```python
from build123d import *

# Parameters (mm, degrees)
BOSS_EXTRUDE1_DEPTH = 0.127
SKETCH2_R           = 3.3782
CUT_EXTRUDE1_DEPTH  = 124.294763186


with BuildPart() as part:
    # Sketch1 → Boss-Extrude1 (new body)
    with BuildSketch(Plane(origin=(0, 0, 0), x_dir=(1, 0, 0), z_dir=(0, 1, 0))):
        with BuildLine():
            Line((19.05, 44.45), (69.85, 44.45))
            ThreePointArc((69.85, 44.45), (74.340128061, 42.590128061), (76.2, 38.1))
            Line((76.2, 38.1), (76.2, -38.1))
            ThreePointArc((76.2, -38.1), (74.340128061, -42.590128061), (69.85, -44.45))
            Line((69.85, -44.45), (19.05, -44.45))
            Line((19.05, -44.45), (19.05, -60.325))
            Line((19.05, -60.325), (15.875, -60.325))
            Line((15.875, -60.325), (15.875, -63.5))
            Line((15.875, -63.5), (19.05, -63.5))
            Line((19.05, -63.5), (19.05, -69.85))
            Line((19.05, -69.85), (69.85, -69.85))
            ThreePointArc((69.85, -69.85), (92.300640303, -60.550640303), (101.6, -38.1))
            Line((101.6, -38.1), (101.6, 38.1))
            ThreePointArc((101.6, 38.1), (92.300640303, 60.550640303), (69.85, 69.85))
            Line((69.85, 69.85), (-69.85, 69.85))
            ThreePointArc((-69.85, 69.85), (-92.300640303, 60.550640303), (-101.6, 38.1))
            Line((-101.6, 38.1), (-101.6, -38.1))
            ThreePointArc((-101.6, -38.1), (-92.300640303, -60.550640303), (-69.85, -69.85))
            Line((-69.85, -69.85), (-19.05, -69.85))
            Line((-19.05, -69.85), (-19.05, -63.5))
            Line((-19.05, -63.5), (-15.875, -63.5))
            Line((-15.875, -63.5), (-15.875, -60.325))
            Line((-15.875, -60.325), (-19.05, -60.325))
            Line((-19.05, -60.325), (-19.05, -44.45))
            Line((-19.05, -44.45), (-69.85, -44.45))
            ThreePointArc((-69.85, -44.45), (-74.340128061, -42.590128061), (-76.2, -38.1))
            Line((-76.2, -38.1), (-76.2, 38.1))
            ThreePointArc((-76.2, 38.1), (-74.340128061, 42.590128061), (-69.85, 44.45))
            Line((-69.85, 44.45), (-19.05, 44.45))
            Line((-19.05, 44.45), (-19.05, 63.5))
            Line((-19.05, 63.5), (19.05, 63.5))
            Line((19.05, 63.5), (19.05, 44.45))
        make_face()
    extrude(amount=BOSS_EXTRUDE1_DEPTH)

    # Sketch2 → Cut-Extrude1 (cut, through all)
    with BuildSketch(Plane(origin=(0, 0.127, 0), x_dir=(1, 0, 0), z_dir=(0, 1, 0))):
        with Locations(Location((-30.48, 61.595, 0), (0, 0, 270))):
            Circle(SKETCH2_R)
        with Locations(Location((-54.61, 61.595, 0), (0, 0, 270))):
            Circle(SKETCH2_R)
        with Locations(Location((30.48, -61.595, 0), (0, 0, 90))):
            Circle(SKETCH2_R)
        with Locations(Location((54.61, -61.595, 0), (0, 0, 90))):
            Circle(SKETCH2_R)
        with Locations(Location((86.463473824, -54.713473824, 0), (0, 0, 90))):
            Circle(SKETCH2_R)
        with Locations(Location((-86.463473824, 54.713473824, 0), (0, 0, 270))):
            Circle(SKETCH2_R)
        with Locations(Location((-93.345, 19.05, 0), (0, 0, 270))):
            Circle(SKETCH2_R)
        with Locations(Location((-93.345, -19.05, 0), (0, 0, 270))):
            Circle(SKETCH2_R)
        with Locations(Location((93.345, -19.05, 0), (0, 0, 90))):
            Circle(SKETCH2_R)
        with Locations(Location((93.345, 19.05, 0), (0, 0, 90))):
            Circle(SKETCH2_R)
        with Locations(Location((86.463473824, 54.713473824, 0), (0, 0, 90))):
            Circle(SKETCH2_R)
        with Locations(Location((-86.463473824, -54.713473824, 0), (0, 0, 270))):
            Circle(SKETCH2_R)
        with Locations(Location((-54.61, -61.595, 0), (0, 0, 270))):
            Circle(SKETCH2_R)
        with Locations(Location((-30.48, -61.595, 0), (0, 0, 270))):
            Circle(SKETCH2_R)
        with Locations(Location((54.61, 61.595, 0), (0, 0, 90))):
            Circle(SKETCH2_R)
        with Locations(Location((30.48, 61.595, 0), (0, 0, 90))):
            Circle(SKETCH2_R)
    extrude(amount=-CUT_EXTRUDE1_DEPTH, mode=Mode.SUBTRACT)


solid = part.part
```
For this review, take the finished solid that the model builds, in its own axes (mm). Coordinates: 2 decimals unless noted, no trailing zeros. Write each loop counter-clockwise with the first axis right and the second up, starting at its lowest first coordinate (ties: lowest second). Pieces come first, ordered by that corner, then holes. Notation, with made-up numbers: (-30, 18.5) -> (5, 18.5) arc R29 cw to (5, 41.5) -> close; hole circle Ø1 at (-25, -31). An arc over 180 degrees is marked (long way). Put each result on its own line as item: value.
Q1. Take a section at B-B, the plane z = 19.05. State the section outline as (x, y) points, then the cut area to 3 significant figures.
From the geometry:
outline: (-101.6, 0) -> (-96.72, 0) -> (-96.72, 0.13) -> (-101.6, 0.13) -> close; (-89.97, 0) -> (-76.2, 0) -> (-76.2, 0.13) -> (-89.97, 0.13) -> close; (76.2, 0) -> (89.97, 0) -> (89.97, 0.13) -> (76.2, 0.13) -> close; (96.72, 0) -> (101.6, 0) -> (101.6, 0.13) -> (96.72, 0.13) -> close
area: 4.74 mm2
Q2. Take a section at D-D, the plane x = -11. State the section outline as (y, z) points.
From the geometry:
outline: (0, -69.85) -> (0.13, -69.85) -> (0.13, -63.5) -> (0, -63.5) -> close
Q3. Wall thickness on L1, parallel to Z at x = 18, y = 0.05 (3 decimals); L2, parallel to X at y = 0.05, z = -3; L3, parallel to X at y = 0.05, z = 46.5: over which ranges is each line inside the solid? List them lowest first.
From the geometry:
L1: z = -69.85 to -63.5, 60.325 to 63.5
L2: x = -101.6 to -76.2, 76.2 to 101.6
L3: x = -100.47 to -19.05, 19.05 to 100.47
Q4. Take a section at C-C, the plane x = -73. State the section outline as (y, z) points.
From the geometry:
outline: (0, -69.69) -> (0.13, -69.69) -> (0.13, -43.61) -> (0, -43.61) -> close; (0, 43.61) -> (0.13, 43.61) -> (0.13, 69.69) -> (0, 69.69) -> close
Q5. Take a section at A-A, the plane x = 54.61. State the section outline as (y, z) points, then the cut area to 3 significant figures.
From the geometry:
outline: (0, -69.85) -> (0.13, -69.85) -> (0.13, -64.97) -> (0, -64.97) -> close; (0, -58.22) -> (0.13, -58.22) -> (0.13, -44.45) -> (0, -44.45) -> close; (0, 44.45) -> (0.13, 44.45) -> (0.13, 58.22) -> (0, 58.22) -> close; (0, 64.97) -> (0.13, 64.97) -> (0.13, 69.85) -> (0, 69.85) -> close
area: 4.74 mm2
